from build123d import *

# Parameters (mm, degrees)
SKETCH_2_W          = 50
SKETCH_2_H          = 105
SKETCH_2_R          = 13.25
SKETCH_2_R_2        = 2.1
EXTRUDE_1_DEPTH     = 3
SKETCH_3_W          = 50
SKETCH_3_H          = 15.05
CUT_EXTRUDE_1_DEPTH = 1
FILLET_1_R          = 5


with BuildPart() as part:
    # ｽｹｯﾁ2 → ﾎﾞｽ - 押し出し1 (new body)
    with BuildSketch(Plane.XY):
        with Locations((25, 52.5)):
            Rectangle(SKETCH_2_W, SKETCH_2_H)
        with Locations((25, 52.5)):
            Circle(SKETCH_2_R, mode=Mode.SUBTRACT)
        with Locations((37.374368671, 64.874368671)):
            Circle(SKETCH_2_R_2, mode=Mode.SUBTRACT)
        with Locations((12.625631329, 64.874368671)):
            Circle(SKETCH_2_R_2, mode=Mode.SUBTRACT)
        with Locations((37.374368671, 40.125631329)):
            Circle(SKETCH_2_R_2, mode=Mode.SUBTRACT)
        with Locations((12.625631329, 40.125631329)):
            Circle(SKETCH_2_R_2, mode=Mode.SUBTRACT)
        with BuildLine():
            Line((5.75, 9.75), (9.25, 9.75))
            ThreePointArc((9.25, 9.75), (11.5, 7.5), (9.25, 5.25))
            Line((9.25, 5.25), (5.75, 5.25))
            ThreePointArc((5.75, 5.25), (3.5, 7.5), (5.75, 9.75))
        make_face(mode=Mode.SUBTRACT)
        with BuildLine():
            Line((40.750000202, 9.75), (44.250000202, 9.75))
            ThreePointArc((44.250000202, 9.75), (46.500000202, 7.5), (44.250000202, 5.25))
            Line((44.250000202, 5.25), (40.750000202, 5.25))
            ThreePointArc((40.750000202, 5.25), (38.500000202, 7.5), (40.750000202, 9.75))
        make_face(mode=Mode.SUBTRACT)
        with BuildLine():
            Line((40.750000101, 99.75), (44.250000101, 99.75))
            ThreePointArc((44.250000101, 99.75), (46.500000101, 97.5), (44.250000101, 95.25))
            Line((44.250000101, 95.25), (40.750000101, 95.25))
            ThreePointArc((40.750000101, 95.25), (38.500000101, 97.5), (40.750000101, 99.75))
        make_face(mode=Mode.SUBTRACT)
        with BuildLine():
            Line((5.749999899, 99.75), (9.249999899, 99.75))
            ThreePointArc((9.249999899, 99.75), (11.499999899, 97.5), (9.249999899, 95.25))
            Line((9.249999899, 95.25), (5.749999899, 95.25))
            ThreePointArc((5.749999899, 95.25), (3.499999899, 97.5), (5.749999899, 99.75))
        make_face(mode=Mode.SUBTRACT)
    extrude(amount=EXTRUDE_1_DEPTH)

    # ｽｹｯﾁ3 → ｶｯﾄ - 押し出し1 (cut)
    with BuildSketch(Plane.XY.offset(3)):
        with Locations((25, 97.475)):
            Rectangle(SKETCH_3_W, SKETCH_3_H)
        with Locations((25, 7.525)):
            Rectangle(SKETCH_3_W, SKETCH_3_H)
    extrude(amount=-CUT_EXTRUDE_1_DEPTH, mode=Mode.SUBTRACT)

    # ﾌｨﾚｯﾄ1
    fillet_1_edges = [part.edges().sort_by_distance(p)[0] for p in [
        (0, 105, 1),
        (50, 105, 1),
        (50, 0, 1),
        (0, 0, 1),
    ]]
    fillet(fillet_1_edges, radius=FILLET_1_R)


solid = part.part
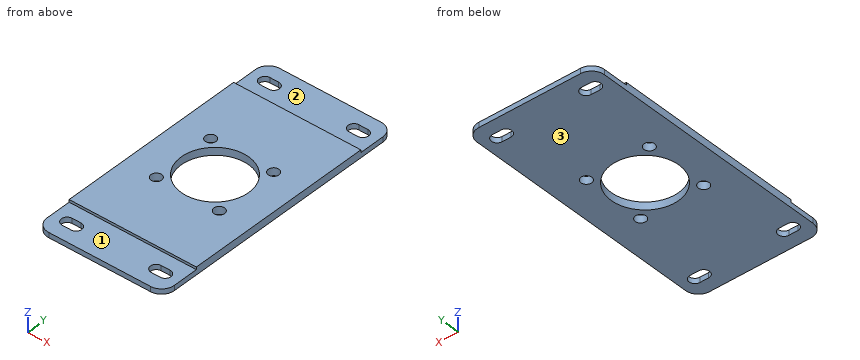
CAD build for the part. Positions are in the model's coordinates, mm. Face numbers are marked on the shaded views. A direction names the side the tool comes from. Coordinates: 2 decimals unless noted, no trailing zeros. Loops run counter-clockwise (first coordinate to the right, second up) from the corner with the lowest first, then second, coordinate; pieces in that order, holes last. Notation, with made-up numbers: (86.5, 22) - (107.5, 22) arc R27 cw to (107.5, 56) - close; hole circle Ø5 at (-35.5, 59). An arc over 180 degrees is marked (long way). Use one line per item in the form item = value. Start each with the question number.
1) Flat gauge pins, fed straight in: pin 1 (16 mm diameter, centred on x = 25, y = 52.5, fed in from -Z); pin 2 (16.5 mm diameter, centred on x = 21, y = 101, fed in from +Z). Where does each tip first touch, or does it go through?
2) Drill centre lines: L1, parallel to Y at x = 7.5, z = 1.4; L2, parallel to Y at x = 13, z = 1.3; L3, parallel to X at y = 38.5, z = 1. Where is each one in solid material? Low to high. Write a range as from..to.
3) Band-saw the part on A-A (x = 25). Give the cut face in (y, z).
4) Band-saw the part on B-B (y = 7.5). Give the cut face in (x, z), and give its area (3 significant figures).
5) Tool access for the marked faces 1, 2 and 3: list every direction of +Z, -Z, +X, -X, +Y, -Y with a clear straight run to the whole face (end or side of a thin tool).
6) Band-saw the part on D-D (z = 0.5). State how many separate pieces and enclosed holes the cut face has, and give its area (3 significant figures).
7) Band-saw the part on C-C (y = 52.5). Give the cut face in (x, z).
Check values:
q1.pin_1 = through
q1.pin_2 = 2
q2.L1 = 0..5.25, 9.75..95.25, 99.75..105
q2.L2 = 0..38.06, 42.19..46.88, 58.12..62.81, 66.94..105
q2.L3 = 0..11.3, 13.96..36.04, 38.7..50
q3.outline = (0, 0) - (39.25, 0) - (39.25, 3) - (15.05, 3) - (15.05, 2) - (0, 2) - close; (65.75, 0) - (105, 0) - (105, 2) - (89.95, 2) - (89.95, 3) - (65.75, 3) - close
q4.outline = (0, 0) - (3.5, 0) - (3.5, 2) - (0, 2) - close; (11.5, 0) - (38.5, 0) - (38.5, 2) - (11.5, 2) - close; (46.5, 0) - (50, 0) - (50, 2) - (46.5, 2) - close
q4.area = 68.0 mm2
q5.face_1 = +Z, +X, -X, -Y
q5.face_2 = +Z, +X, -X, +Y
q5.face_3 = -Z, +X, -X, +Y, -Y
q6.separate_pieces = 1
q6.enclosed_holes = 9
q6.area = 4,490 mm2
q7.outline = (0, 0) - (11.75, 0) - (11.75, 3) - (0, 3) - close; (38.25, 0) - (50, 0) - (50, 3) - (38.25, 3) - close
